```python
from build123d import *

# Parameters (mm, degrees)
SKETCH1_W               = 76
SKETCH1_H               = 44
BOSS_EXTRUDE1_DEPTH     = 38
SKETCH2_R               = 7.5
CUT_EXTRUDE1_DEPTH      = 1
CUT_EXTRUDE1_DEPTH_BACK = 45
SKETCH3_W               = 22.449944321
SKETCH3_H               = 32
SKETCH3_W_2             = 32.550055679
SKETCH3_H_2             = 22
CUT_EXTRUDE2_DEPTH      = 1
CUT_EXTRUDE2_DEPTH_BACK = 39
SKETCH5_W               = 44
SKETCH5_H               = 38
SKETCH4_W               = 21
SKETCH4_H               = 21
SKETCH6_R               = 5.5
CUT_EXTRUDE3_DEPTH      = 1.0000001
CUT_EXTRUDE3_DEPTH_BACK = 102


with BuildPart() as part:
    # Sketch1 → Boss-Extrude1 (new body)
    with BuildSketch(Plane(origin=(0, 0, 0), x_dir=(1, 0, 0), z_dir=(0, 1, 0))):
        Rectangle(SKETCH1_W, SKETCH1_H)
    extrude(amount=BOSS_EXTRUDE1_DEPTH)

    # Sketch2 → Cut-Extrude1 (cut, two sides)
    with BuildSketch(Plane.XY.offset(22)) as cut_extrude1_sk:
        with Locations((-15.550055679, 13)):
            Circle(SKETCH2_R)
        with BuildLine():
            Line((-15.550055679, 38), (-38, 38))
            Line((-38, 38), (-38, 24))
            ThreePointArc((-38, 24), (-28.778812235, 34.213203436), (-15.550055679, 38))
        make_face()
    extrude(amount=CUT_EXTRUDE1_DEPTH, mode=Mode.SUBTRACT)
    extrude(cut_extrude1_sk.sketch, amount=-CUT_EXTRUDE1_DEPTH_BACK, mode=Mode.SUBTRACT)

    # Sketch3 → Cut-Extrude2 (cut, two sides)
    with BuildSketch(Plane(origin=(0, 38, 0), x_dir=(1, 0, 0), z_dir=(0, 1, 0))) as cut_extrude2_sk:
        with Locations((-26.77502784, 0)):
            Rectangle(SKETCH3_W, SKETCH3_H)
        with Locations((0.72497216, 0)):
            Rectangle(SKETCH3_W_2, SKETCH3_H_2)
    extrude(amount=CUT_EXTRUDE2_DEPTH, mode=Mode.SUBTRACT)
    extrude(cut_extrude2_sk.sketch, amount=-CUT_EXTRUDE2_DEPTH_BACK, mode=Mode.SUBTRACT)

    # Sketch5 → Loft1 section 0
    with BuildSketch(Plane(origin=(38, 0, 0), x_dir=(0, 0, -1), z_dir=(1, 0, 0))):
        with Locations((0, 19)):
            Rectangle(SKETCH5_W, SKETCH5_H)
    # Sketch4 → Loft1 section 1
    with BuildSketch(Plane(origin=(63, 0, 0), x_dir=(0, 0, -1), z_dir=(1, 0, 0))):
        with Locations((0, 19)):
            Rectangle(SKETCH4_W, SKETCH4_H)
    loft()

    # Sketch6 → Cut-Extrude3 (cut, two sides)
    with BuildSketch(Plane(origin=(63, 0, 0), x_dir=(0, 0, -1), z_dir=(1, 0, 0))) as cut_extrude3_sk:
        with Locations((0, 19)):
            Circle(SKETCH6_R)
    extrude(amount=CUT_EXTRUDE3_DEPTH, mode=Mode.SUBTRACT)
    extrude(cut_extrude3_sk.sketch, amount=-CUT_EXTRUDE3_DEPTH_BACK, mode=Mode.SUBTRACT)


solid = part.part
```
Geometry: final body of the model. Coordinates: model frame, mm. A direction names the side the tool comes from. Give positions to 0.01 mm unless a question says otherwise; leave off trailing zeros. Write each loop counter-clockwise with the first axis right and the second up, starting at its lowest first coordinate (ties: lowest second). Pieces come first, ordered by that corner, then holes.
1. Draft query along Z for faces 1 (the cylindrical face through (40.322, 24.453, 0.716)), 2 (the flat face through (-1, 19, -22)), 3 (the flat face through (25, 0, 0)), 4 (the flat face through (17, 15, 5)). Return one class per face: released by +Z, released by -Z, zero draft, split by the parting line, or undercut.
2. Reachability of faces 5 (the cylindrical face through (-8.62, 10.13, 17.8)), 6 (the flat face through (-15.55, 3, -13)) from +Z, -Z, +X, -X, +Y, -Y: full face, straight path, thin tool, end or side. Return the list, or none.
3. Section query A-A, the plane x = 6.5. Return loops of the section in (y, z), then the cut area to 3 significant figures.
4. Line query: probe 1 along Z at (x, y) = (8, 30.5); probe 2 along Y at (x, z) = (28, 0); probe 3 along Z at (x, y) = (-27.5, 7). Output: solid intervals per line, ascending.
5. Pin query (flat end, axial travel): P1, Ø17.5, axis at y = 15, z = 0, coming from the -X side; P2, Ø1.5, axis at x = 42.5, z = -14.5, coming from the +Y side (3 decimals); P3, Ø1.5, axis at y = 29, z = 13, coming from the -X side. Return the tip coordinate at first contact, or that it passes through.
6. Section query B-B, the plane y = 11. Count the separate pieces of the cut face and the enclosed holes in it, then the cut area to 3 significant figures.
Computed:
1. face 1: undercut
1. face 2: released by -Z
1. face 3: zero draft
1. face 4: undercut
2. face 5: +Z, -Z
2. face 6: -X, +Y, -Y
3. outline: (0, -22) - (38, -22) - (38, -11) - (0, -11) - close; (0, 11) - (38, 11) - (38, 22) - (0, 22) - close
3. area: 836 mm2
4. probe 1: z = -22 to -11, 11 to 22
4. probe 2: y = 0 to 13.5, 24.5 to 38
4. probe 3: z = -22 to -16, 16 to 22
5. P1: stops at x = 17
5. P2: stops at y = 36.725
5. P3: stops at x = -15.55
6. separate pieces: 3
6. enclosed holes: 0
6. area: 2,480 mm2
